The model under review builds one solid part; all positions refer to its coordinate system, in mm. A direction names the side the tool comes from. Coordinates: 2 decimals unless noted, no trailing zeros. Order: outer loops, then holes, each group sorted by start corner. A loop starts at its lowest first (then second) coordinate and runs counter-clockwise, first axis right, second up. Notation, with made-up numbers: M 25,37.25 L 83,37.25 A20 cw 83,44.25 Z; hole C 21,21.25 d2. An arc over 180 degrees is marked long. Answer as CSV lines item,"result". Start each with the question number.
Q1. Wall thickness on L1, parallel to Z at x = 6, y = 560.5: over which ranges is the line inside the solid? List them lowest first. Write a range as [from, to].
Q2. Consider section A-A on z = 7.5. Write out the cut boundary in (x, y).
Q3. For P1, Ø10, axis at x = -19.5, z = -9, coming from the +Y side, flat-tipped, find the tip position at first contact; note if it passes through.
Q4. The part is to be moulded in two halves that separate along X. For faces 1 (the face through (25.4, 351, 0)), 2 (the face through (-2.166, 17.132, -26.361)), 3 (the face through (0, 351, 27.508)), 4 (the face through (0, 351, 25.4)), say which applies: +X half, -X half, draft (parallel to the pull), parting line (faces both ways), or undercut.
Q5. Machinability: for faces 5 (the face through (-27.508, 351, 0)), 6 (the face through (-25.4, 351, 0)), which of the approach directions +Z, -Z, +X, -X, +Y, -Y give a long, thin tool a straight path to every point of the face, cutting with its end or side? Answer none if there is none.
Q6. Consider section C-C on y = 432. Write out the cut boundary in (x, z).
Q7. Consider section B-B on x = -18. Write out the cut boundary in (y, z).
Autodesk Inventor part; units mm, degrees
ref_plane "YZ Plane" through (0, 0, 0) normal (1, 0, 0) x (0, 1, 0)
ref_plane "XZ Plane" through (0, 0, 0) normal (0, 1, 0) x (-1, 0, 0)
ref_plane "XY Plane" through (0, 0, 0) normal (0, 0, 1) x (1, 0, 0)
sketch "Sketch1" plane through (0, 0, 0) normal (0, 1, 0) x (-1, 0, 0)
  line L0 (25.4, 25.4) -> (-25.4, 25.4)
  line L1 (-25.4, 25.4) -> (-25.4, -25.4)
  line L2 (-25.4, -25.4) -> (25.4, -25.4)
  line L3 (25.4, -25.4) -> (25.4, 25.4)
  line L4 (-27.5082, 27.5082) -> (27.5082, 27.5082)
  line L5 (27.5082, 27.5082) -> (27.5082, -27.5082)
  line L6 (27.5082, -27.5082) -> (-27.5082, -27.5082)
  line L7 (-27.5082, -27.5082) -> (-27.5082, 27.5082)
  point P0 (0, 0)
  point P1 (25.4, 0)
  point P2 (0, -25.4)
  dimension "d0" = 50.8
  dimension "d1" = 50.8
  dimension "d2" = 2.1082
extrude "Extrusion1" add sketch "Sketch1" along normal blind 711.2
sketch "Sketch2" plane through (-27.5082, 0, 27.5082) normal (0, 0, 1) x (1, 0, 0)
  line L0 (0, 0) -> (55.0164, 0)
  line L1 (55.0164, 0) -> (0, 0)
  line L2 (0, 31.7637) -> (55.0164, 0)
  line L3 (0, 0) -> (0, 711.2)
  line L4 (0, 31.7637) -> (0, 0)
  line L5 (2.1082, 0) -> (2.1082, 711.2)
  line L6 (0, 711.2) -> (55.0164, 711.2)
  line L7 (0, 711.2) -> (55.0164, 711.2)
  line L8 (55.0164, 711.2) -> (0, 679.4363)
  line L9 (0, 679.4363) -> (0, 711.2)
  point P0 (27.5082, 0)
  dimension "d5" = 30
  dimension "d6" = 30
extrude "Extrusion2" cut sketch "Sketch2" against normal through all contours L3 L2 L5 L0 | L5 L2 L0 | L3 L6 L5 L8 | L5 L6 L8
properties part number "Square_30degree"
Evaluation:
1,L1,"z = [-27.51, -25.4], [25.4, 27.51]"
2,outline,"M -27.51,31.76 L -25.4,30.55 L -25.4,680.65 L -27.51,679.44 Z; M 25.4,1.22 L 27.51,0 L 27.51,711.2 L 25.4,709.98 Z"
3,P1,"passes through"
4,face 1,"undercut"
4,face 2,"-X half"
4,face 3,"draft"
4,face 4,"undercut"
5,face 5,"+Z, -Z, -X, +Y, -Y"
5,face 6,"+Y, -Y"
6,outline,"M -27.51,-27.51 L 27.51,-27.51 L 27.51,27.51 L -27.51,27.51 Z; hole M -25.4,-25.4 L 25.4,-25.4 L 25.4,25.4 L -25.4,25.4 Z"
7,outline,"M 26.27,-27.51 L 684.93,-27.51 L 684.93,-25.4 L 26.27,-25.4 Z; M 26.27,25.4 L 684.93,25.4 L 684.93,27.51 L 26.27,27.51 Z"
